Build history of the part. All positions in model axes, mm. A direction names the side the tool comes from. Give positions to 0.01 mm unless a question says otherwise; leave off trailing zeros. Write each loop counter-clockwise with the first axis right and the second up, starting at its lowest first coordinate (ties: lowest second). Pieces come first, ordered by that corner, then holes. Notation, with made-up numbers: (70.5, -1.5) -> (89.5, -1.5) arc R24 ccw to (89.5, 20.5) -> close; hole circle Ø1 at (1.25, -29). An arc over 180 degrees is marked (long way). Put each result on its own line as item: value.
from build123d import *

# Parameters (mm, degrees)
SKETCH2_R           = 2.1
CUT_EXTRUDE1_DEPTH  = 6
CIRPATTERN1_COUNT   = 6
CUT_EXTRUDE2_REACH  = 108.536
SKETCH3_R           = 4.4
CIRPATTERN2_COUNT   = 10
BOSS_EXTRUDE1_START = 10
SKETCH4_R           = 5.5
BOSS_EXTRUDE1_DEPTH = 10
SKETCH5_R           = 5.5
CUT_EXTRUDE3_DEPTH  = 3
CUT_EXTRUDE4_REACH  = 108.86
SKETCH6_R           = 1


with BuildPart() as part:
    # Sketch1 → Revolve1 (revolve)
    with BuildSketch(Plane.XY, mode=Mode.PRIVATE) as revolve1_sk:
        Polygon((0, 12), (17, 12), (17, 53), (20, 53), (20, 55), (16.9, 55), (16.9, 60.4), (20, 60.4), (20, 75), (10, 75), (10, 24), (0, 24), align=None)
    revolve(revolve1_sk.sketch.rotate(Axis((0, 0, 0), (1, 0, 0)), 90), axis=Axis((0, 0, 0), (1, 0, 0)))

    # Sketch2 → Cut-Extrude1 (cut)
    with BuildSketch(Plane.ZY):
        with Locations((0, 18)):
            Circle(SKETCH2_R)
    cut_extrude1 = extrude(amount=-CUT_EXTRUDE1_DEPTH, mode=Mode.SUBTRACT)

    # CirPattern1: Cut-Extrude1 ×6 about axis
    cirpattern1_axis = Axis((0, 0, 0), (1, 0, 0))
    for i in range(1, CIRPATTERN1_COUNT):
        add(cut_extrude1.rotate(cirpattern1_axis, i * 360 / CIRPATTERN1_COUNT), mode=Mode.SUBTRACT)

    # Sketch3 → Cut-Extrude2 (cut, up to next)
    with BuildSketch(Plane.ZY.offset(-10), mode=Mode.PRIVATE) as cut_extrude2_sk1:
        with Locations((0, 67)):
            Circle(SKETCH3_R)
    cut_extrude2_tool1 = extrude(cut_extrude2_sk1.sketch, amount=-CUT_EXTRUDE2_REACH, mode=Mode.PRIVATE) & part.part
    cut_extrude2 = cut_extrude2_tool1.solids().sort_by_distance((10, 67, 0))[0]
    add(cut_extrude2, mode=Mode.SUBTRACT)

    # CirPattern2: Cut-Extrude2 ×10 about axis
    cirpattern2_axis = Axis((0, 0, 0), (1, 0, 0))
    for i in range(1, CIRPATTERN2_COUNT):
        add(cut_extrude2.rotate(cirpattern2_axis, i * 360 / CIRPATTERN2_COUNT), mode=Mode.SUBTRACT)

    # Sketch4 → Boss-Extrude1 (add)
    with BuildSketch(Plane.ZY.offset(-10).offset(BOSS_EXTRUDE1_START)):
        with BuildLine():
            Line((-21.84352517, 9.942857143), (-8.64639538, 38.935714286))
            ThreePointArc((-8.64639538, 38.935714286), (0, 44.5), (8.64639538, 38.935714286))
            Line((8.64639538, 38.935714286), (21.84352517, 9.942857143))
            ThreePointArc((21.84352517, 9.942857143), (0, 24), (-21.84352517, 9.942857143))
        make_face()
        with Locations((0, 35)):
            Circle(SKETCH4_R, mode=Mode.SUBTRACT)
    extrude(amount=-BOSS_EXTRUDE1_DEPTH)

    # Sketch5 → Cut-Extrude3 (cut)
    with BuildSketch(Plane.ZY.offset(-10)):
        with Locations((0, 35)):
            Circle(SKETCH5_R)
    extrude(amount=-CUT_EXTRUDE3_DEPTH, mode=Mode.SUBTRACT)

    # Sketch6 → Cut-Extrude4 (cut, up to next)
    with BuildSketch(Plane.ZY.offset(-13), mode=Mode.PRIVATE) as cut_extrude4_sk1:
        with Locations((0, 35)):
            Circle(SKETCH6_R)
    cut_extrude4_tool1 = extrude(cut_extrude4_sk1.sketch, amount=-CUT_EXTRUDE4_REACH, mode=Mode.PRIVATE) & part.part
    add(cut_extrude4_tool1.solids().sort_by_distance((13, 35, 0))[0], mode=Mode.SUBTRACT)


solid = part.part
1) Slice it at A-A (x = 1.75). Give the number of separate pieces and of enclosed holes in the cut face, plus the area to 3 significant figures.
Filled sheet:
separate pieces: 1
enclosed holes: 8
area: 1,690 mm2
2) Wall check: L1, parallel to Y at x = 17.6, z = 0; L2, parallel to Z at x = 15.75, y = 55; L3, parallel to Y at x = 18.25, z = -38. Give the ranges that are in metal, low to high.
Filled sheet:
L1: -75 to -71.4, -62.6 to -60.4, -55 to -53, 53 to 55, 60.4 to 62.6, 71.4 to 75
L2: -50.99 to -43.71, -35.05 to 35.05, 43.71 to 50.99
L3: -64.66 to -58.38, -50.03 to -46.95, -39.76 to -36.95, 36.95 to 39.76, 46.95 to 50.03, 58.38 to 64.66
3) Tool access for faces 1 (the cylindrical face through (18.52, -52.55, -6.9)), 2 (the flat face through (6, -9, 16)), 3 (the flat face through (20, 61, 0)): list every direction of +Z, -Z, +X, -X, +Y, -Y with a clear straight run to the whole face (end or side of a thin tool).
Filled sheet:
face 1: +X
face 2: -X
face 3: +Z, -Z, +X, +Y, -Y
4) Slice it at C-C (y = -14). Write the cut outline in (x, z).
Filled sheet:
outline: (0, -19.49) -> (10, -19.49) -> (10, -73.68) -> (20, -73.68) -> (20, -58.76) -> (16.9, -58.76) -> (16.9, -53.19) -> (20, -53.19) -> (20, -51.12) -> (17, -51.12) -> (17, 51.12) -> (20, 51.12) -> (20, 53.19) -> (16.9, 53.19) -> (16.9, 58.76) -> (20, 58.76) -> (20, 73.68) -> (10, 73.68) -> (10, 19.49) -> (0, 19.49) -> close
5) Pin check, flat tips, straight feed: pin 1 (3 mm diameter, centred on x = 10.5, y = -53.5, fed in from -Z); pin 2 (6 mm diameter, centred on x = 8.5, y = 9, fed in from -Z); pin 3 (2.5 mm diameter, centred on y = -18, z = 0, fed in from -X). Stop position of each tip, or through.
Filled sheet:
pin 1: z = -54.05
pin 2: z = -74.73
pin 3: x = 6
6) Slice it at B-B (z = -47). Write the cut outline in (x, y).
Filled sheet:
outline: (10, -58.45) -> (20, -58.45) -> (20, -37.94) -> (16.9, -37.94) -> (16.9, -28.57) -> (20, -28.57) -> (20, -24.49) -> (17, -24.49) -> (17, 24.49) -> (20, 24.49) -> (20, 28.57) -> (16.9, 28.57) -> (16.9, 37.94) -> (20, 37.94) -> (20, 58.45) -> (10, 58.45) -> close
7) Pull direction Z, two halves, no side cores. Call faces 4 (the flat face through (0, 10, -11)), 5 (the cylindrical face through (14.93, 66.538, 34.608)), 6 (the flat face through (6, 9, -16)), 7 (the cylindrical face through (14.93, -22.6, -67.69)): released by +Z, released by -Z, zero draft, split by the parting line, or undercut.
Filled sheet:
face 4: zero draft
face 5: split by the parting line
face 6: undercut
face 7: undercut
